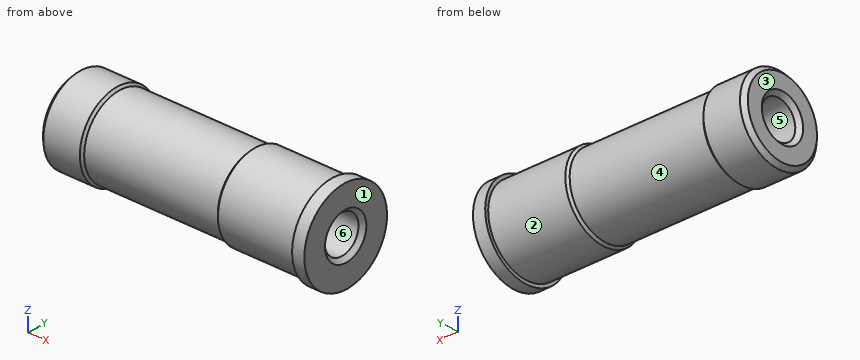
from build123d import *

# Parameters (mm, degrees)
SFAZOWANIE1_SIZE = 1
SFAZOWANIE2_SIZE = 1
SFAZOWANIE3_SIZE = 1


with BuildPart() as part:
    # Szkic1 → Obrót1 (revolve)
    with BuildSketch(Plane.XY, mode=Mode.PRIVATE) as obr_t1_sk:
        Polygon((0, 4.5), (0, 10.2), (11, 10.2), (11, 9.65), (43, 9.65), (43, 10.2), (63, 10.2), (63, 11), (66, 11), (66, 4.5), (42, 4.5), (42, 0), (19, 0), (19, 4.5), align=None)
    revolve(obr_t1_sk.sketch.rotate(Axis((0, 0, 0), (1, 0, 0)), 90), axis=Axis((0, 0, 0), (1, 0, 0)))

    # Sfazowanie1
    sfazowanie1_edges = [part.edges().sort_by_distance(p)[0] for p in [
        (0, 0, -10.2),
    ]]
    chamfer(sfazowanie1_edges, length=SFAZOWANIE1_SIZE)

    # Sfazowanie2
    # the kernel refuses this chamfer: 1 mm, written as the material it takes off along each edge
    with BuildSketch(Plane(origin=(11, 0, 0), x_dir=(0, 0, 1), z_dir=(0, 1, 0))) as sfazowanie2_piece_1_section:
        Polygon((10.2, -SFAZOWANIE2_SIZE), (10.2 - SFAZOWANIE2_SIZE, 0), (10.2, 0), align=None)
    sfazowanie2_piece_1 = revolve(axis=Axis((11, 0, 0), (1, 0, 0)), mode=Mode.PRIVATE)
    sfazowanie2_piece_1 = sfazowanie2_piece_1 - Plane(origin=(10.282118865, 0, 0), x_dir=(0, 0, 1), z_dir=(1, 0, 0)) * Cylinder(9.65, 41, mode=Mode.PRIVATE)
    add(sfazowanie2_piece_1, mode=Mode.SUBTRACT)
    with BuildSketch(Plane(origin=(43, 0, 0), x_dir=(0, 0, 1), z_dir=(0, 1, 0))) as sfazowanie2_piece_2_section:
        Polygon((10.2 - SFAZOWANIE2_SIZE, 0), (10.2, SFAZOWANIE2_SIZE), (10.2, 0), align=None)
    sfazowanie2_piece_2 = revolve(axis=Axis((43, 0, 0), (1, 0, 0)), mode=Mode.PRIVATE)
    sfazowanie2_piece_2 = sfazowanie2_piece_2 - Plane(origin=(43.717881135, 0, 0), x_dir=(0, 0, 1), z_dir=(1, 0, 0)) * Cylinder(9.65, 41, mode=Mode.PRIVATE)
    add(sfazowanie2_piece_2, mode=Mode.SUBTRACT)

    # Sfazowanie3
    sfazowanie3_edges = [part.edges().sort_by_distance(p)[0] for p in [
        (0, 0, -4.5),
        (66, 0, -4.5),
    ]]
    chamfer(sfazowanie3_edges, length=SFAZOWANIE3_SIZE)


solid = part.part
Design review of the part built by this model. Coordinates are the model's own, in mm. Face numbers are marked on the shaded views. A direction names the side the tool comes from. Give positions to 0.01 mm unless a question says otherwise; leave off trailing zeros. Order: outer loops, then holes, each group sorted by start corner. A loop starts at its lowest first (then second) coordinate and runs counter-clockwise, first axis right, second up.
1. Mouldability with a two-part tool opening along Y and no side actions: class the marked faces 3, 4, 5 and 6 as +Y half, -Y half, draft (parallel to the pull), parting line (faces both ways), or undercut.
Solution:
face 3: draft
face 4: parting line
face 5: undercut
face 6: undercut
2. For pin 1 Ø5 at (y, z) = (-1, 0) entering from -X; pin 2 Ø4 at (x, y) = (7.5, 0) entering from +Z; pin 3 Ø3 at (x, z) = (17, -8) entering from +Y, all flat-tipped, find the tip position at first contact; note any pin that passes through.
Solution:
pin 1: stops at x = 19
pin 2: stops at z = 10.2
pin 3: stops at y = 7.13
3. Add section B-B, the plane x = 45.5. State the section outline as (y, z) points, then the cut area to 3 significant figures.
Solution:
outline: circle Ø20.4 at (0, 0); hole circle Ø9 at (0, 0)
area: 263 mm2
4. To check wall thickness, follow L1, parallel to Y at x = 10.75, z = 0; L2, parallel to X at y = -0.5, z = -3.75; L3, parallel to Z at x = 9, y = -1.75. State the ranges of each line that lie inside material, in increasing order.
Solution:
L1: y = -9.65 to -4.5, 4.5 to 9.65
L2: x = 19 to 42
L3: z = -10.05 to -4.15, 4.15 to 10.05
5. Tool access review of the marked faces 1 and 2: name each direction out of +Z, -Z, +X, -X, +Y, -Y from which nothing blocks a thin tool from reaching the whole face with its end or side.
Solution:
face 1: +Z, -Z, +X, +Y, -Y
face 2: -X
